Source: CAD feature listing. Evaluate the final solid. Frame: model axes, mm. A direction names the side the tool comes from. Give positions to 0.01 mm unless a question says otherwise; leave off trailing zeros. Order: outer loops, then holes, each group sorted by start corner. A loop starts at its lowest first (then second) coordinate and runs counter-clockwise, first axis right, second up.
```python
from build123d import *

# Parameters (mm, degrees)
BASE_FLANGE1_DEPTH     = 6
SKETCHED_START         = -25
SKETCHED_BEND1_DEPTH   = 50
SKETCHED_BEND1_2_DEPTH = 50
SKETCH7_R              = 1.5
CUT_EXTRUDE1_DEPTH     = 92.073510938
FILLET1_R              = 5
SKETCH8_R              = 3
CUT_EXTRUDE2_DEPTH     = 97.955579492


# Read off the part's stored shape, not the designer's step: Sketched Bend1
# Sheet-metal steps are written as plain solids
with BuildPart() as part:
    # Sketch1 → Base-Flange1 (new body)
    with BuildSketch(Plane(origin=(0, 0, 0), x_dir=(1, 0, 0), z_dir=(0, 1, 0))):
        Polygon((25, 20), (79, 20), (79, -20), (-79, -20), (-79, 20), (-25, 20), (-25, 60), (25, 60), align=None)
    extrude(amount=-BASE_FLANGE1_DEPTH)

    # Sketched Bend1 outline → Sketched Bend1 (cut)
    with BuildSketch(Plane.YZ.offset(SKETCHED_START)):
        with BuildLine():
            Line((0, -60), (0, -30.677078252))
            ThreePointArc((0, -30.677078252), (-4.397247359, -26.123724357), (-6, -20))
            Line((-6, -20), (-6, -60))
            Line((-6, -60), (0, -60))
        make_face()
    extrude(amount=SKETCHED_BEND1_DEPTH, mode=Mode.SUBTRACT)

    # Sketched Bend1 2 outline → Sketched Bend1 2 (add)
    with BuildSketch(Plane.YZ.offset(SKETCHED_START)):
        with BuildLine():
            Line((6.5, -32.5), (31.577434895, -32.5))
            Line((31.577434895, -32.5), (31.577434895, -26.5))
            Line((31.577434895, -26.5), (6.5, -26.5))
            ThreePointArc((6.5, -26.5), (1.903805922, -24.596194078), (0, -20))
            Line((0, -20), (0, -30.677078252))
            ThreePointArc((0, -30.677078252), (3.124609515, -32.035644523), (6.5, -32.5))
        make_face()
    extrude(amount=SKETCHED_BEND1_2_DEPTH)

    # Sketch7 → Cut-Extrude1 (cut, through all)
    with BuildSketch(Plane(origin=(0, 0, 0), x_dir=(1, 0, 0), z_dir=(0, 1, 0))):
        with Locations(Location((-70, -7, 0), (0, 0, 270))):
            Circle(SKETCH7_R)
        with Locations(Location((-70, -14, 0), (0, 0, 270))):
            Circle(SKETCH7_R)
        with Locations(Location((70, -14, 0), (0, 0, 90))):
            Circle(SKETCH7_R)
        with Locations(Location((70, -7, 0), (0, 0, 90))):
            Circle(SKETCH7_R)
    extrude(amount=-CUT_EXTRUDE1_DEPTH, mode=Mode.SUBTRACT)

    # Fillet1
    fillet1_edges = [part.edges().sort_by_distance(p)[0] for p in [
        (-79, -3, 20),
        (79, -3, 20),
        (79, -3, -20),
        (-79, -3, -20),
    ]]
    fillet(fillet1_edges, radius=FILLET1_R)

    # Sketch8 → Cut-Extrude2 (cut, through all)
    with BuildSketch(Plane.XY.offset(-26.5)):
        with Locations((-7.5, 21.577434895)):
            Circle(SKETCH8_R)
        with Locations(Location((7.5, 21.577434895, 0), (0, 0, 180))):
            Circle(SKETCH8_R)
    extrude(amount=-CUT_EXTRUDE2_DEPTH, mode=Mode.SUBTRACT)


solid = part.part
```
1) Section query B-B, the plane x = -7.5. Return the cut outline in (y, z).
Report:
outline: (-6, -20) arc R12.5 ccw to (6.5, -32.5) - (18.58, -32.5) - (18.58, -26.5) - (6.5, -26.5) arc R6.5 cw to (0, -20) - (0, 20) - (-6, 20) - close; (24.58, -32.5) - (31.58, -32.5) - (31.58, -26.5) - (24.58, -26.5) - close
2) Pin query (flat end, axial travel): pin 1 (20 mm diameter, centred on x = 12, z = 8, fed in from +Y); pin 2 (6 mm diameter, centred on x = 20, y = 12.5, fed in from +Z); pin 3 (3 mm diameter, centred on x = 47.5, y = -1.5, fed in from -Z). Return the tip coordinate at first contact, or that it passes through.
Report:
pin 1: stops at y = 0
pin 2: stops at z = -26.5
pin 3: stops at z = -20
3) Reachability of faces 1 (the flat face through (1, 0, 0)), 2 (the flat face through (49, -3, -20)), 3 (the cylindrical face through (-77, -3, -19)) from +Z, -Z, +X, -X, +Y, -Y: full face, straight path, thin tool, end or side. Return the list, or none.
Report:
face 1: +Z, +X, -X, +Y
face 2: -Z, +X, +Y, -Y
face 3: -Z, -X, +Y, -Y
4) Section query A-A, the plane x = 70. Return the cut outline in (y, z).
Report:
outline: (-6, -20) - (0, -20) - (0, 5.5) - (-6, 5.5) - close; (-6, 8.5) - (0, 8.5) - (0, 12.5) - (-6, 12.5) - close; (-6, 15.5) - (0, 15.5) - (0, 20) - (-6, 20) - close
5) Section query C-C, the plane z = 7. Return the cut outline in (x, y), and give its area (3 significant figures).
Report:
outline: (-79, -6) - (-71.5, -6) - (-71.5, 0) - (-79, 0) - close; (-68.5, -6) - (68.5, -6) - (68.5, 0) - (-68.5, 0) - close; (71.5, -6) - (79, -6) - (79, 0) - (71.5, 0) - close
area: 912 mm2
6) Section query D-D, the plane z = -28. Return the cut outline in (x, y).
Report:
outline: (-25, -3.1) - (25, -3.1) - (25, 31.58) - (-25, 31.58) - close; hole circle Ø6 at (-7.5, 21.58); hole circle Ø6 at (7.5, 21.58)
7) Draft query along X for faces 4 (the flat face through (-25, 13, -28)), 5 (the cylindrical face through (77, -3, -19)), 6 (the cylindrical face through (6.12, 24.24, -29.46)). Return one class per face: +X half, -X half, draft (parallel to the pull), parting line (faces both ways), or undercut.
Report:
face 4: -X half
face 5: +X half
face 6: undercut
8) Material intervals for L1, parallel to X at y = -1.85, z = 7; L2, parallel to Y at x = 13, z = 5.5; L3, parallel to Z at x = 16, y = 10.5, sorted ascending.
Report:
L1: x = -79 to -71.5, -68.5 to 68.5, 71.5 to 79
L2: y = -6 to 0
L3: z = -32.5 to -26.5
